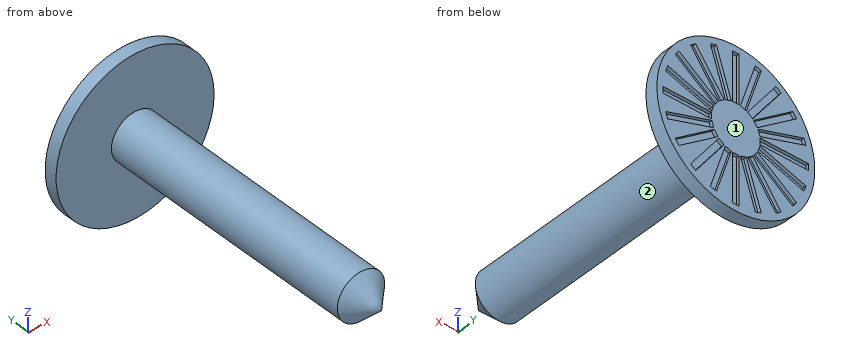
from build123d import *

# Parameters (mm, degrees)
F0_R            = 12.5
F1_DEPTH        = 2
F2_R            = 3.75
F3_DEPTH        = 45
F4_SIZE         = 3.75
F7_DEPTH        = 0.5
F7_COPIES_COUNT = 20


# Not quite as in the source:
# - a pattern or mirror of a feature is missing from the dataset's text; its kind, count and spacing are read off the source's solid


with BuildPart() as f1:
    # F0 (on Front) → F1 (new body)
    with BuildSketch(Plane.XZ):
        Circle(F0_R)
    extrude(amount=F1_DEPTH)

    # F2 (on face) → F3 (join)
    with BuildSketch(Plane.XZ.offset(2)):
        Circle(F2_R)
    extrude(amount=F3_DEPTH)

    # F4
    f4_edges = [f1.edges().sort_by_distance(p)[0] for p in [
        (-3.75, -47, 0),
    ]]
    chamfer(f4_edges, length=F4_SIZE)

    # F6 (on Front) → F7 (cut)
    with BuildSketch(Plane.XZ):
        with BuildLine():
            Line((-0.5, 3.85), (0.5, 3.85))
            Line((0.5, 3.85), (0.5, 11.4891252931))
            ThreePointArc((0.5, 11.4891252931), (0, 11.5), (-0.5, 11.4891252931))
            Line((-0.5, 11.4891252931), (-0.5, 3.85))
        make_face()
    f7 = extrude(amount=F7_DEPTH, mode=Mode.SUBTRACT)

    # F7_copies: F7 ×20 about axis
    f7_copies_axis = Axis((0, 0, 0), (0, 1, 0))
    for i in range(1, F7_COPIES_COUNT):
        add(f7.rotate(f7_copies_axis, i * 360 / F7_COPIES_COUNT), mode=Mode.SUBTRACT)


solid = f1.part
Model file for the job. Use its own axes, mm. Face numbers are marked on the shaded views. A direction names the side the tool comes from. Round coordinates to 2 decimals unless told otherwise and drop trailing zeros. Loops run counter-clockwise (first coordinate to the right, second up) from the corner with the lowest first, then second, coordinate; pieces in that order, holes last. Notation, with made-up numbers: (-27.5, -38) - (-7.5, -38) arc R21 ccw to (-7.5, -34) - close; hole circle Ø2 at (-6.5, -22.5). An arc over 180 degrees is marked (long way). Write each question's results on one line, items separated by ' | '.
(1) Wall check: L1, parallel to Y at x = 8.75, z = 4; L2, parallel to Y at x = -7.75, z = -2.25; L3, parallel to X at y = -22, z = -0.25. Give the ranges that are in metal, low to high.
Answer below:
L1: y = -2 to 0 | L2: y = -2 to -0.5 | L3: x = -3.74 to 3.74
(2) Pin check, flat tips, straight feed: pin 1 (4 mm diameter, centred on x = 2.5, z = 2.5, fed in from -Y); pin 2 (3 mm diameter, centred on y = -25.5, z = 4, fed in from +X); pin 3 (0.5 mm diameter, centred on x = 0, z = -7.5, fed in from +Y). Stop position of each tip, or through.
Answer below:
pin 1: stops at y = -45.46 | pin 2: stops at x = 2.8 | pin 3: stops at y = -0.5
(3) Saw through at B-B, the plane y = -42.5. List the corners of the cut face in (x, z), then the cut area to 3 significant figures.
Answer below:
outline: circle Ø7.5 at (0, 0) | area: 44.2 mm^2
(4) Saw through at A-A, the plane z = -8.5. List the corners of the cut face in (x, y).
Answer below:
outline: (-9.17, -2) - (9.17, -2) - (9.17, 0) - (6.79, 0) - (6.79, -0.5) - (5.56, -0.5) - (5.56, 0) - (3.29, 0) - (3.29, -0.5) - (2.24, -0.5) - (2.24, 0) - (0.5, 0) - (0.5, -0.5) - (-0.5, -0.5) - (-0.5, 0) - (-2.24, 0) - (-2.24, -0.5) - (-3.29, -0.5) - (-3.29, 0) - (-5.56, 0) - (-5.56, -0.5) - (-6.79, -0.5) - (-6.79, 0) - (-9.17, 0) - close
(5) 3-axis set-ups, long thin cutter, end or side, ignore diameter. For the marked faces 1 and 2: which of +Z, -Z, +X, -X, +Y, -Y reach the whole face in a straight line?
Answer below:
face 1: +Z, -Z, +X, -X, +Y | face 2: -Y
